Source: three-view drawing plus pictorial views. Frame: mm from the lowest corner of the part. A direction names the side the tool comes from. Round coordinates to 2 decimals unless told otherwise and drop trailing zeros. Loops run counter-clockwise (first coordinate to the right, second up) from the corner with the lowest first, then second, coordinate; pieces in that order, holes last. Notation, with made-up numbers: (80, -22) -> (94, -22) arc R28 cw to (94, -4) -> close; hole circle Ø10 at (-6, 61.5). An arc over 180 degrees is marked (long way). Answer in a Markdown table with one row per item.
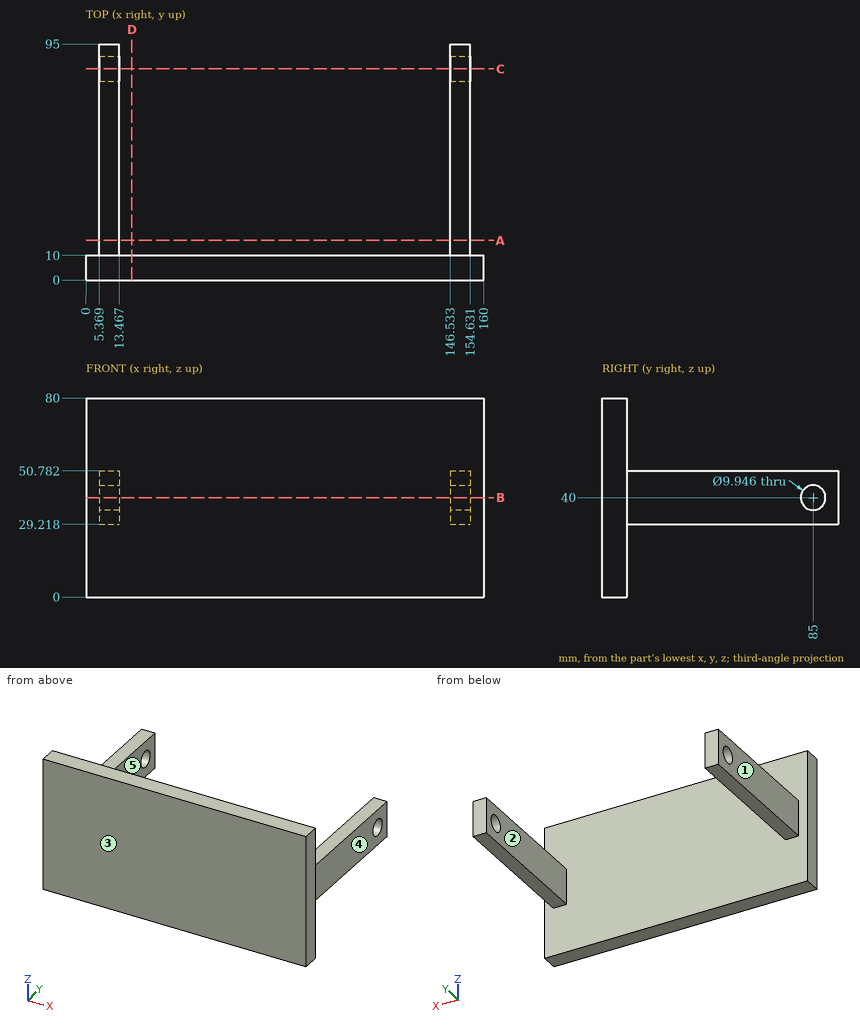
Item 1: Cut plane A-A (y = 16). Output: boundary loops of the cut face in (x, z).
Answer:
| item | result |
|---|---|
| outline | (5.37, 29.22) -> (13.47, 29.22) -> (13.47, 50.78) -> (5.37, 50.78) -> close; (146.53, 29.22) -> (154.63, 29.22) -> (154.63, 50.78) -> (146.53, 50.78) -> close |
Item 2: Reachability of the marked faces 1 and 2 from +Z, -Z, +X, -X, +Y, -Y: full face, straight path, thin tool, end or side. Return the list, or none.
Answer:
| item | result |
|---|---|
| face 1 | +Z, -Z, -X, +Y |
| face 2 | +Z, -Z, +Y |
Item 3: Cut plane D-D (x = 18.5). Output: boundary loops of the cut face in (y, z), then the cut area to 3 significant figures.
Answer:
| item | result |
|---|---|
| outline | (0, 0) -> (10, 0) -> (10, 80) -> (0, 80) -> close |
| area | 800 mm² |
Item 4: Cut plane C-C (y = 85). Output: boundary loops of the cut face in (x, z), then the cut area to 3 significant figures.
Answer:
| item | result |
|---|---|
| outline | (5.37, 29.22) -> (13.47, 29.22) -> (13.47, 35.03) -> (5.37, 35.03) -> close; (5.37, 44.97) -> (13.47, 44.97) -> (13.47, 50.78) -> (5.37, 50.78) -> close; (146.53, 29.22) -> (154.63, 29.22) -> (154.63, 35.03) -> (146.53, 35.03) -> close; (146.53, 44.97) -> (154.63, 44.97) -> (154.63, 50.78) -> (146.53, 50.78) -> close |
| area | 188 mm² |
Item 5: Draft query along X for the marked faces 3, 4 and 5. Return one class per face: pulls with the +X half, pulls with the -X half, needs draft (parallel to the pull), parting line crosses it, or undercut.
Answer:
| item | result |
|---|---|
| face 3 | needs draft |
| face 4 | pulls with the +X half |
| face 5 | undercut |
Item 6: Pin query (flat end, axial travel): pin 1 Ø4 at (y, z) = (63, 40) entering from -X; pin 2 Ø23.5 at (y, z) = (58, 38.5) entering from +X; pin 3 Ø12 at (x, z) = (117.5, 36) entering from +Y. Return the tip coordinate at first contact, or that it passes through.
Answer:
| item | result |
|---|---|
| pin 1 | stops at x = 5.37 |
| pin 2 | stops at x = 154.63 |
| pin 3 | stops at y = 10 |
Item 7: Line query: probe 1 along Y at (x, z) = (9.25, 40); probe 2 along X at (y, z) = (36.5, 44.5); probe 3 along Y at (x, z) = (103, 31.5). Output: solid intervals per line, ascending. Write a range as [from, to].
Answer:
| item | result |
|---|---|
| probe 1 | y = [0, 80.03], [89.97, 95] |
| probe 2 | x = [5.37, 13.47], [146.53, 154.63] |
| probe 3 | y = [0, 10] |
Item 8: Cut plane B-B (z = 40). Output: boundary loops of the cut face in (x, y).
Answer:
| item | result |
|---|---|
| outline | (0, 0) -> (160, 0) -> (160, 10) -> (154.63, 10) -> (154.63, 80.03) -> (146.53, 80.03) -> (146.53, 10) -> (13.47, 10) -> (13.47, 80.03) -> (5.37, 80.03) -> (5.37, 10) -> (0, 10) -> close; (5.37, 89.97) -> (13.47, 89.97) -> (13.47, 95) -> (5.37, 95) -> close; (146.53, 89.97) -> (154.63, 89.97) -> (154.63, 95) -> (146.53, 95) -> close |
